from build123d import *

# Parameters (mm, degrees)
SKETCH1_R           = 2.1828125
BOSS_EXTRUDE1_DEPTH = 6.35
CHAMFER1_SIZE       = 0.396875


with BuildPart() as part:
    # Sketch1 → Boss-Extrude1 (new body)
    with BuildSketch(Plane(origin=(0, 0, 0), x_dir=(1, 0, 0), z_dir=(0, 1, 0))):
        with BuildLine():
            Line((6.35, 25.4), (6.35, 0))
            ThreePointArc((6.35, 0), (5.492179091, -3.187235296), (3.150482259, -5.513343952))
            Line((3.150482259, -5.513343952), (-19.074517741, -18.213343952))
            ThreePointArc((-19.074517741, -18.213343952), (-23.067855509, -18.993813994), (-26.715128061, -17.190128061))
            Line((-26.715128061, -17.190128061), (-52.115128061, 8.209871939))
            ThreePointArc((-52.115128061, 8.209871939), (-53.491635031, 15.130039796), (-47.625, 19.05))
            Line((-47.625, 19.05), (-17.960512242, 19.05))
            ThreePointArc((-17.960512242, 19.05), (-15.530472447, 19.533364969), (-13.470384182, 20.909871939))
            Line((-13.470384182, 20.909871939), (-4.490128061, 29.890128061))
            ThreePointArc((-4.490128061, 29.890128061), (2.430039796, 31.266635031), (6.35, 25.4))
        make_face()
        Circle(SKETCH1_R, mode=Mode.SUBTRACT)
        with Locations((0, 25.4)):
            Circle(SKETCH1_R, mode=Mode.SUBTRACT)
        with Locations((-22.225, 0)):
            Circle(SKETCH1_R, mode=Mode.SUBTRACT)
        with Locations((-22.225, -12.7)):
            Circle(SKETCH1_R, mode=Mode.SUBTRACT)
        with Locations((-34.925, 12.7)):
            Circle(SKETCH1_R, mode=Mode.SUBTRACT)
        with Locations((-47.625, 12.7)):
            Circle(SKETCH1_R, mode=Mode.SUBTRACT)
    extrude(amount=BOSS_EXTRUDE1_DEPTH)

    # Chamfer1
    chamfer1_edges = [part.edges().sort_by_distance(p)[0] for p in [
        (-32.792756121, 0, -19.05),
        (-15.530472447, 0, -19.533364969),
        (-8.980256121, 0, -25.4),
        (2.430039796, 0, -31.266635031),
        (6.35, 0, -12.7),
        (5.492179091, 0, 3.187235296),
        (-7.962017741, 0, 11.863343952),
        (-23.067855509, 6.35, 18.993813994),
        (-23.067855509, 0, 18.993813994),
        (-39.415128061, 0, 4.490128061),
        (-53.491635031, 0, -15.130039796),
        (-7.962017741, 6.35, 11.863343952),
        (5.492179091, 6.35, 3.187235296),
        (6.35, 6.35, -12.7),
        (-2.1828125, 0, 0),
        (-2.1828125, 6.35, 0),
        (2.430039796, 6.35, -31.266635031),
        (-2.1828125, 0, -25.4),
        (-2.1828125, 6.35, -25.4),
        (-8.980256121, 6.35, -25.4),
        (-24.4078125, 0, 0),
        (-24.4078125, 6.35, 0),
        (-15.530472447, 6.35, -19.533364969),
        (-24.4078125, 0, 12.7),
        (-24.4078125, 6.35, 12.7),
        (-32.792756121, 6.35, -19.05),
        (-37.1078125, 0, -12.7),
        (-37.1078125, 6.35, -12.7),
        (-49.8078125, 0, -12.7),
        (-49.8078125, 6.35, -12.7),
        (-53.491635031, 6.35, -15.130039796),
        (-39.415128061, 6.35, 4.490128061),
    ]]
    chamfer(chamfer1_edges, length=CHAMFER1_SIZE)


solid = part.part
Build history of the part. All positions in model axes, mm. Give positions to 0.01 mm unless a question says otherwise; leave off trailing zeros. Order: outer loops, then holes, each group sorted by start corner. A loop starts at its lowest first (then second) coordinate and runs counter-clockwise, first axis right, second up. Notation, with made-up numbers: M -37,-29.75 L 22,-29.75 A17 cw 22,-2.75 Z; hole C -37,39 d9. An arc over 180 degrees is marked long. Put each result on its own line as item: value.
Item 1: Wall check: probe 1 along X at (y, z) = (3.4, -12.7) (3 decimals); probe 2 along X at (y, z) = (1.8, 0); probe 3 along Z at (x, y) = (0, 3.5). Give the ranges that are in metal, low to high.
Results are:
probe 1: -53.975 to -49.808, -45.442 to -37.108, -32.742 to 6.35
probe 2: -43.91 to -24.41, -20.04 to -2.18, 2.18 to 6.35
probe 3: -31.75 to -27.58, -23.22 to -2.18, 2.18 to 7.31
Item 2: Cut at A-A on z = -12.7. Write the cut outline in (x, y) (3 decimals), then the cut area to 3 significant figures.
Results are:
outline: M -53.975,0.397 L -53.578,0 L -50.205,0 L -49.808,0.397 L -49.808,5.953 L -50.205,6.35 L -53.578,6.35 L -53.975,5.953 Z; M -45.442,0.397 L -45.045,0 L -37.505,0 L -37.108,0.397 L -37.108,5.953 L -37.505,6.35 L -45.045,6.35 L -45.442,5.953 Z; M -32.742,0.397 L -32.345,0 L 5.953,0 L 6.35,0.397 L 6.35,5.953 L 5.953,6.35 L -32.345,6.35 L -32.742,5.953 Z
area: 327 mm2
Item 3: Cut at D-D on x = 0. Write the cut outline in (y, z), then the cut area to 3 significant figures.
Results are:
outline: M 0,-31.35 L 0.4,-31.75 L 5.95,-31.75 L 6.35,-31.35 L 6.35,-27.98 L 5.95,-27.58 L 0.4,-27.58 L 0,-27.98 Z; M 0,-22.82 L 0.4,-23.22 L 5.95,-23.22 L 6.35,-22.82 L 6.35,-2.58 L 5.95,-2.18 L 0.4,-2.18 L 0,-2.58 Z; M 0,2.58 L 0.4,2.18 L 5.95,2.18 L 6.35,2.58 L 6.35,6.86 L 5.95,7.31 L 0.4,7.31 L 0,6.86 Z
area: 192 mm2
Item 4: Cut at C-C on z = 12.7. Write the cut outline in (x, y), then the cut area to 3 significant figures.
Results are:
outline: M -31.21,0.4 L -30.64,0 L -24.8,0 L -24.41,0.4 L -24.41,5.95 L -24.8,6.35 L -30.64,6.35 L -31.21,5.95 Z; M -20.04,0.4 L -19.65,0 L -10.23,0 L -9.43,0.4 L -9.43,5.95 L -10.23,6.35 L -19.65,6.35 L -20.04,5.95 Z
area: 110 mm2
Item 5: Cut at B-B on y = 4.5. Write the cut outline in (x, z) (3 decimals).
Results are:
outline: M -52.115,-8.21 A6.35 ccw -47.625,-19.05 L -17.961,-19.05 A6.35 cw -13.47,-20.91 L -4.49,-29.89 A6.35 ccw 6.35,-25.4 L 6.35,0 A6.35 ccw 3.15,5.513 L -19.075,18.213 A6.35 ccw -26.715,17.19 Z; hole C -47.625,-12.7 d4.366; hole C -34.925,-12.7 d4.366; hole C -22.225,0 d4.366; hole C -22.225,12.7 d4.366; hole C 0,-25.4 d4.366; hole C 0,0 d4.366
Item 6: Pull direction Z, two halves, no side cores. Call faces 1 (the face through (-24.406, 3.136, 12.604)), 2 (the face through (-7.906, 6.154, 11.6)), 3 (the face through (-9.04, 3.14, -25.34)), 4 (the face through (-49.806, 3.136, -12.796)): +Z half, -Z half, draft (parallel to the pull), parting line (faces both ways), or undercut.
Results are:
face 1: undercut
face 2: +Z half
face 3: -Z half
face 4: undercut
Item 7: Drop flat-ended pins along their axis: pin 1 Ø4 at (x, z) = (-22.225, 12.7) entering from +Y; pin 2 Ø5 at (x, z) = (-22.225, 0) entering from +Y. Give the stop position or say it passes through.
Results are:
pin 1: through
pin 2: y = 6.27
